```python
from build123d import *

# Parameters (mm, degrees)
SKETCH2_W           = 78
SKETCH2_H           = 10
BOSS_EXTRUDE1_DEPTH = 3.175
SKETCH3_R           = 2.5
CUT_EXTRUDE1_DEPTH  = 3.175
CUT_EXTRUDE2_REACH  = 41.447
SKETCH4_R           = 1


with BuildPart() as part:
    # Sketch2 → Boss-Extrude1 (new body)
    with BuildSketch(Plane(origin=(0, 0, 0), x_dir=(1, 0, 0), z_dir=(0, 1, 0))):
        Rectangle(SKETCH2_W, SKETCH2_H)
    extrude(amount=BOSS_EXTRUDE1_DEPTH)

    # Sketch3 → Cut-Extrude1 (cut)
    with BuildSketch(Plane(origin=(0, 3.175, 0), x_dir=(1, 0, 0), z_dir=(0, 1, 0))):
        with Locations(Location((-34, 0, 0), (0, 0, 270))):
            Circle(SKETCH3_R)
        with Locations(Location((34, 0, 0), (0, 0, 90))):
            Circle(SKETCH3_R)
    extrude(amount=-CUT_EXTRUDE1_DEPTH, mode=Mode.SUBTRACT)

    # Sketch4 → Cut-Extrude2 (cut, up to next)
    with BuildSketch(Plane(origin=(0, 3.175, 0), x_dir=(1, 0, 0), z_dir=(0, 1, 0)), mode=Mode.PRIVATE) as cut_extrude2_sk1:
        with Locations(Location((-19.5, 0, 0), (0, 0, 270))):
            Circle(SKETCH4_R)
    cut_extrude2_tool1 = extrude(cut_extrude2_sk1.sketch, amount=-CUT_EXTRUDE2_REACH, mode=Mode.PRIVATE) & part.part
    add(cut_extrude2_tool1.solids().sort_by_distance((-19.5, 3.175, 0))[0], mode=Mode.SUBTRACT)


solid = part.part
```
Geometry: final body of the model. Coordinates: model frame, mm. Give positions to 0.01 mm unless a question says otherwise; leave off trailing zeros. Loops run counter-clockwise (first coordinate to the right, second up) from the corner with the lowest first, then second, coordinate; pieces in that order, holes last. Notation, with made-up numbers: (61, 79) -> (108, 79) arc R10 ccw to (108, 83) -> close; hole circle Ø2 at (-5, 27.25). An arc over 180 degrees is marked (long way). Return JSON: item names as keys, results as strings.
Item 1: Pin query (flat end, axial travel): P1, Ø1.2, axis at x = -19.5, z = 0, coming from the -Y side; P2, Ø4, axis at x = 20.5, z = 1.5, coming from the -Y side. Return the tip coordinate at first contact, or that it passes through.
Filled in:
{"P1": "through", "P2": "y = 0"}
Item 2: Line query: line 1 (X direction, y = 1, z = 0); line 2 (Z direction, x = 34, y = 2.35); line 3 (X direction, y = 1.4, z = -1.75). Output: solid intervals per line, ascending.
Filled in:
{"line 1": "-39 to -36.5, -31.5 to -20.5, -18.5 to 31.5, 36.5 to 39", "line 2": "-5 to -2.5, 2.5 to 5", "line 3": "-39 to -35.79, -32.21 to 32.21, 35.79 to 39"}
Item 3: Section D-D, the plane x = 34. Output: boundary loops of the cut face in (y, z) (3 decimals).
Filled in:
{"outline": "(0, -5) -> (3.175, -5) -> (3.175, -2.5) -> (0, -2.5) -> close; (0, 2.5) -> (3.175, 2.5) -> (3.175, 5) -> (0, 5) -> close"}
Item 4: Section B-B, the plane z = 0. Output: boundary loops of the cut face in (x, y) (3 decimals).
Filled in:
{"outline": "(-39, 0) -> (-36.5, 0) -> (-36.5, 3.175) -> (-39, 3.175) -> close; (-31.5, 0) -> (-20.5, 0) -> (-20.5, 3.175) -> (-31.5, 3.175) -> close; (-18.5, 0) -> (31.5, 0) -> (31.5, 3.175) -> (-18.5, 3.175) -> close; (36.5, 0) -> (39, 0) -> (39, 3.175) -> (36.5, 3.175) -> close"}
Item 5: Section A-A, the plane x = -19.5. Output: boundary loops of the cut face in (y, z) (3 decimals).
Filled in:
{"outline": "(0, -5) -> (3.175, -5) -> (3.175, -1) -> (0, -1) -> close; (0, 1) -> (3.175, 1) -> (3.175, 5) -> (0, 5) -> close"}
Item 6: Section C-C, the plane y = 0.7. Output: boundary loops of the cut face in (x, z), plus the area to 3 significant figures.
Filled in:
{"outline": "(-39, -5) -> (39, -5) -> (39, 5) -> (-39, 5) -> close; hole circle Ø5 at (-34, 0); hole circle Ø2 at (-19.5, 0); hole circle Ø5 at (34, 0)", "area": "738 mm^2"}
Item 7: Mould query, pull axis X, two halves, no side actions, for faces 1 (the flat face through (-1, 0, 0)), 2 (the flat face through (39, 2, 0)), 3 (the cylindrical face through (-31.52, 1.61, -0.33)), 4 (the cylindrical face through (-20.476, 1.61, -0.217)). Classes: released by +X, released by -X, zero draft, split by the parting line, or undercut.
Filled in:
{"face 1": "zero draft", "face 2": "released by +X", "face 3": "undercut", "face 4": "undercut"}
